For this review, take the finished solid that the model builds, in its own axes (mm). Face numbers are marked on the shaded views. A direction names the side the tool comes from. Give positions to 0.01 mm unless a question says otherwise; leave off trailing zeros. Loops run counter-clockwise (first coordinate to the right, second up) from the corner with the lowest first, then second, coordinate; pieces in that order, holes last. Notation, with made-up numbers: M -15.5,88.5 L 37.5,88.5 A26 ccw 37.5,126.5 Z; hole C -12.75,76.5 d8. An arc over 180 degrees is marked long. Use CSV: the item, a comma, the result in double quotes. Start each with the question number.
1. The part is to be moulded in two halves that separate along Z. For the marked faces 3 and 4, say which applies: pulls with the +Z half, pulls with the -Z half, needs draft (parallel to the pull), parting line crosses it, or undercut.
2. Tool access review of the marked faces 1 and 2: name each direction out of +Z, -Z, +X, -X, +Y, -Y from which nothing blocks a thin tool from reaching the whole face with its end or side.
3. To check wall thickness, follow line 1 (Z direction, x = 0, y = 0.45); line 2 (Z direction, x = 0, y = 2.9); line 3 (Y direction, x = 1, z = -3.5). State the ranges of each line that lie inside material, in increasing order. Write a range as [from, to].
4. Take a section at A-A, the plane y = 2.2. Write out the cut boundary in (x, z).
5. Insertion check: P1, Ø1, axis at x = 4.5, y = 1, coming from the -Z side; P2, Ø2.5, axis at x = 0, z = 0, coming from the -Y side. Each pin has a flat end and moves straight along its axis. Give the tip position at first contact, or say it passes through.
Autodesk Inventor part; units mm, degrees
ref_plane "YZ Plane" through (0, 0, 0) normal (1, 0, 0) x (0, 1, 0)
ref_plane "XZ Plane" through (0, 0, 0) normal (0, 1, 0) x (-1, 0, 0)
ref_plane "XY Plane" through (0, 0, 0) normal (0, 0, 1) x (1, 0, 0)
sketch "Эскиз1" plane through (0, 0, 0) normal (0, 1, 0) x (-1, 0, 0)
  circle A0 centre (0, 0) radius 6.5
  circle A1 centre (0, 0) radius 2
  dimension "d0" = 13
  dimension "d1" = 4
extrude "Выдавливание1" add sketch "Эскиз1" along normal blind 5
sketch "Эскиз2" plane through (0, 5, 0) normal (0, 1, 0) x (1, 0, 0)
  circle A0 centre (0, 0) radius 3
  circle A1 centre (0, 0) radius 5.5
  circle A2 centre (0, 0) radius 6.5
  circle A3 centre (0, 0) radius 2
  dimension "d4" = 1
  dimension "d5" = 1
extrude "Выдавливание2" cut sketch "Эскиз2" against normal blind 0.5 contours A1
sketch "Эскиз3" plane through (0, 0, 0) normal (0, -1, 0) x (1, 0, 0)
  circle A0 centre (0, 0) radius 3
  circle A1 centre (0, 0) radius 5.5
extrude "Выдавливание3" cut sketch "Эскиз3" against normal blind 0.5
chamfer "Фаска1" distance 0.2 angle 45 8 edges at (-3, 0, 0) (2, 0, 0) (-5.5, 0, 0) (6.5, 0, 0) (6.5, 5, 0) (-5.5, 5, 0) (-3, 5, 0) (2, 5, 0)
properties part number "Подшипник 626Z" material "Титан"
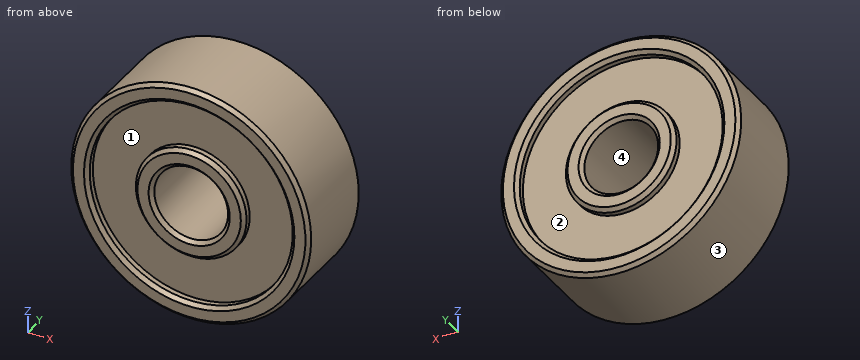
Result set:
1,face 3,"parting line crosses it"
1,face 4,"undercut"
2,face 1,"-Y"
2,face 2,"+Y"
3,line 1,"[-6.5, -5.5], [-3, -2], [2, 3], [5.5, 6.5]"
3,line 2,"[-6.5, -2], [2, 6.5]"
3,line 3,"[0.5, 4.5]"
4,outline,"C 0,0 d13; hole C 0,0 d4"
5,P1,"z = -5.12"
5,P2,"through"
